For this review, take the finished solid that the model builds, in its own axes (mm). Give positions to 0.01 mm unless a question says otherwise; leave off trailing zeros. Write each loop counter-clockwise with the first axis right and the second up, starting at its lowest first coordinate (ties: lowest second). Pieces come first, ordered by that corner, then holes. Notation, with made-up numbers: M -21,-0.75 L -3,-0.75 A13 cw -3,6.25 Z; hole C -38,38.5 d4. An arc over 180 degrees is marked long. One line per item, written item: value. Start each with the question number.
Item 1: Consider section B-B, the plane x = 1463. Write out the cut boundary in (y, z) (3 decimals).
Item 2: Mouldability with a two-part tool opening along X and no side actions: class faces 1 (the face through (1120.709, -1571.768, 6.261)), 2 (the face through (1062.07, -1565.66, 7.92)), 3 (the face through (1314, -1315, 0)) as released by +X, released by -X, zero draft, split by the parting line, or undercut.
Item 3: Consider section A-A, the plane y = -1750. Write out the cut boundary in (x, z).
Item 4: To check wall thickness, follow probe 1 along Y at (x, z) = (718, 6.75); probe 2 along X at (y, z) = (-1078, 9.25); probe 3 along X at (y, z) = (-1224.5, 3.75) (3 decimals). State the ranges of each line that lie inside material, in increasing order.
Item 5: Clearance check with flat-ended pins moving along their axes: pin 1 Ø1.5 at (y, z) = (-1391, 5.5) entering from +X; pin 2 Ø2 at (y, z) = (-1426, 5) entering from +X; pin 3 Ø6 at (x, z) = (1084, 5) entering from -Y. State where each tip first meets the part, or that it passes through.
Solid Edge part; units mm, degrees
sketch "Sketch1" plane through (0, 0, 0) normal (0, 0, 1) x (1, 0, 0)
  line L0 (524.9437, -191.5504) -> (1813.8262, -660.6653)
  line L1 (0.4572, -1930.4) -> (0.4572, -558.7998)
  arc A0 (1813.8262, -660.6653) -> (0.4572, -1930.4) centre (-0.0001, 0) cw
  arc A1 (524.9437, -191.5504) -> (0.4572, -558.7998) centre (0, 0) cw
  circle A2 centre (713.8732, -1019.5166) radius 647.7
extrude "Protrusion1" add sketch "Sketch1" along normal blind 12.7
chamfer "Chamfer_1" distance 3.175 angle 45 1 edges at (66.1732, -1019.5166, 12.7)
chamfer "Chamfer_2" distance 6.35 angle 45 1 edges at (66.1732, -1019.5166, 0)
Model answer:
1. outline: M -1259.395,0 L -532.975,0 L -532.975,12.7 L -1259.395,12.7 Z
2. face 1: released by +X
2. face 2: undercut
2. face 3: zero draft
3. outline: M 0.46,0 L 814.83,0 L 814.83,12.7 L 0.46,12.7 Z
4. probe 1: y = -1791.9 to -1667.2, -371.83 to -261.82
4. probe 2: x = 0.46 to 68.82, 1358.93 to 1601.36
4. probe 3: x = 0.457 to 96.725, 1331.021 to 1492.328
5. pin 1: stops at x = 1339.27
5. pin 2: stops at x = 1302.24
5. pin 3: stops at y = -1599.34
